from build123d import *

# Parameters (mm, degrees)
SKETCH1_R                 = 5
SKETCH1_R_2               = 3.5
BOSS_EXTRUDE1_DEPTH       = 2
SKETCH2_R                 = 11
SKETCH2_R_2               = 4
BOSS_EXTRUDE2_DEPTH       = 1.25
SKETCH2_2_R               = 11
SKETCH2_2_R_2             = 4
BOSS_EXTRUDE3_DEPTH       = 0.75
SKETCH3_R                 = 5
SKETCH3_R_2               = 4
BOSS_EXTRUDE4_DEPTH       = 2.25
M2X0_4_TAPPED_HOLE1_D     = 1.6
M2X0_4_TAPPED_HOLE1_DEPTH = 5.2
M2X0_4_TAPPED_HOLE1_TIP   = 0.480688495


with BuildPart() as part:
    # Sketch1 → Boss-Extrude1 (new body)
    with BuildSketch(Plane(origin=(0, 0, 0), x_dir=(0, 0, -1), z_dir=(1, 0, 0))):
        Circle(SKETCH1_R)
        Circle(SKETCH1_R_2, mode=Mode.SUBTRACT)
    extrude(amount=BOSS_EXTRUDE1_DEPTH)

    # Sketch2 → Boss-Extrude2 (add)
    with BuildSketch(Plane(origin=(2, 0, 0), x_dir=(0, 0, -1), z_dir=(1, 0, 0))):
        Circle(SKETCH2_R)
        Circle(SKETCH2_R_2, mode=Mode.SUBTRACT)
    extrude(amount=BOSS_EXTRUDE2_DEPTH)

    # Sketch2_2 → Boss-Extrude3 (add)
    with BuildSketch(Plane(origin=(2, 0, 0), x_dir=(0, 0, -1), z_dir=(1, 0, 0))):
        Circle(SKETCH2_2_R)
        Circle(SKETCH2_2_R_2, mode=Mode.SUBTRACT)
    extrude(amount=-BOSS_EXTRUDE3_DEPTH)

    # Sketch3 → Boss-Extrude4 (add)
    with BuildSketch(Plane(origin=(3.25, 0, 0), x_dir=(0, 0, -1), z_dir=(1, 0, 0))):
        Circle(SKETCH3_R)
        Circle(SKETCH3_R_2, mode=Mode.SUBTRACT)
    extrude(amount=BOSS_EXTRUDE4_DEPTH)

    # M2x0.4 Tapped Hole1
    with Locations(Plane(origin=(3.25, 0, 0), x_dir=(0, 0, -1), z_dir=(1, 0, 0))):
        with Locations((8, 0), (0, 8), (-5.656854249, 5.656854249), (5.656854249, 5.656854249), (5.656854249, -5.656854249), (0, -8), (-5.656854249, -5.656854249), (-8, 0)):
            Hole(M2X0_4_TAPPED_HOLE1_D / 2, depth=M2X0_4_TAPPED_HOLE1_DEPTH)
            with Locations((0, 0, -(M2X0_4_TAPPED_HOLE1_DEPTH + M2X0_4_TAPPED_HOLE1_TIP / 2))):  # 118° drill point
                Cone(0, M2X0_4_TAPPED_HOLE1_D / 2, M2X0_4_TAPPED_HOLE1_TIP, mode=Mode.SUBTRACT)


solid = part.part
Geometry: final body of the model. Coordinates: model frame, mm. A direction names the side the tool comes from. Give positions to 0.01 mm unless a question says otherwise; leave off trailing zeros. Loops run counter-clockwise (first coordinate to the right, second up) from the corner with the lowest first, then second, coordinate; pieces in that order, holes last. Notation, with made-up numbers: M -2.75,-13 L 48.25,-13 A25 ccw 48.25,5 Z; hole C 66.25,75 d11. An arc over 180 degrees is marked long. Put each result on its own line as item: value.
1) Mould query, pull axis Y, two halves, no side actions, for faces 1 (the flat face through (3.25, -2, -5)), 2 (the cylindrical face through (4.36, -4.88, 1.08)), 3 (the cylindrical face through (2.24, -5.42, 6.42)). Classes: released by +Y, released by -Y, zero draft, split by the parting line, or undercut.
Computed values:
face 1: zero draft
face 2: split by the parting line
face 3: undercut
2) Reachability of faces 4 (the cylindrical face through (2.236, -5.622, -6.456)), 5 (the flat face through (1.25, -2, -5)), 6 (the cylindrical face through (3.726, -3.905, 0.867)) from +Z, -Z, +X, -X, +Y, -Y: full face, straight path, thin tool, end or side. Return the list, or none.
Computed values:
face 4: +X, -X
face 5: -X
face 6: +X
3) Material intervals for L1, parallel to Y at x = 2.75, z = 0; L2, parallel to Y at x = 1.35, z = 0; L3, parallel to X at y = 8.5, z = -5.25, sorted ascending. Write a range as from..to.
Computed values:
L1: y = -11..-8.8, -7.2..-4, 4..7.2, 8.8..11
L2: y = -11..-8.8, -7.2..-3.5, 3.5..7.2, 8.8..11
L3: x = 1.25..3.25
4) Cut plane A-A, the plane z = 0. Return the cut outline in (x, y), plus the area to 3 significant figures.
Computed values:
outline: M 0,-5 L 1.25,-5 L 1.25,-7.2 L 3.25,-7.2 L 3.25,-5 L 5.5,-5 L 5.5,-4 L 2,-4 L 2,-3.5 L 0,-3.5 Z; M 0,3.5 L 2,3.5 L 2,4 L 5.5,4 L 5.5,5 L 3.25,5 L 3.25,7.2 L 1.25,7.2 L 1.25,5 L 0,5 Z; M 1.25,-11 L 3.25,-11 L 3.25,-8.8 L 1.25,-8.8 Z; M 1.25,8.8 L 3.25,8.8 L 3.25,11 L 1.25,11 Z
area: 30.6 mm^2
5) First-contact query: P1, Ø3, axis at y = 5.5, z = 5, coming from the -X side; P2, Ø1.4, axis at y = -5.66, z = -5.66, coming from the +X side; P3, Ø2, axis at y = -5.5, z = 7.5, coming from the +X side; P4, Ø2.5, axis at y = -2, z = 1.5, coming from the +X side. Flat tips, straight axial feed; report the tip coordinate or a pass-through.
Computed values:
P1: stops at x = 1.25
P2: passes through
P3: stops at x = 3.25
P4: stops at x = 2
6) Cut plane D-D, the plane z = -5.75. Return the cut outline in (x, y), plus the area to 3 significant figures.
Computed values:
outline: M 1.25,-9.38 L 3.25,-9.38 L 3.25,-6.45 L 1.25,-6.45 Z; M 1.25,-4.86 L 3.25,-4.86 L 3.25,4.86 L 1.25,4.86 Z; M 1.25,6.45 L 3.25,6.45 L 3.25,9.38 L 1.25,9.38 Z
area: 31.2 mm^2
7) Cut plane C-C, the plane x = 2.6. Give the number of separate pieces and of enclosed holes in the cut face, plus the area to 3 significant figures.
Computed values:
separate pieces: 1
enclosed holes: 9
area: 314 mm^2
